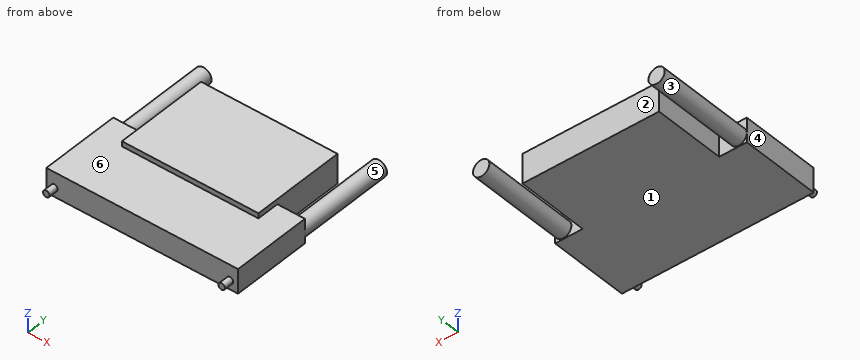
```python
from build123d import *

# Parameters (mm, degrees)
F0_W     = 41.8
F0_H     = 22
F1_DEPTH = 7.45
F2_W     = 41.8
F2_H     = 28.9
F3_DEPTH = 1.55
F4_R     = 1
F5_DEPTH = 3
F6_R     = 2.5
F7_DEPTH = 30


with BuildPart() as f1:
    # F0 (on Top) → F1 (new body)
    with BuildSketch(Plane.XY):
        Polygon((-29.35, 0), (29.35, 0), (29.35, 24.44), (20.9, 24.44), (-20.9, 24.44), (-29.35, 24.44), align=None)
        with Locations((0, 35.44)):
            Rectangle(F0_W, F0_H)
    extrude(amount=F1_DEPTH)

    # F2 (on face) → F3 (join)
    with BuildSketch(Plane.XY.offset(7.45)):
        with Locations((0, 31.99)):
            Rectangle(F2_W, F2_H)
    extrude(amount=F3_DEPTH)

    # F4 (on face) → F5 (join)
    with BuildSketch(Plane.XZ):
        with Locations((-26.85, 2.78)):
            Circle(F4_R)
        with Locations((26.85, 2.78)):
            Circle(F4_R)
    extrude(amount=F5_DEPTH)

    # F6 (on face) → F7 (join)
    with BuildSketch(Plane(origin=(0, 24.44, 0), x_dir=(-1, 0, 0), z_dir=(0, 1, 0))):
        with Locations((-26.85, 2.78)):
            Circle(F6_R)
        with Locations((26.85, 2.78)):
            Circle(F6_R)
    extrude(amount=F7_DEPTH)


solid = f1.part
```
Model file for the job. Use its own axes, mm. Face numbers are marked on the shaded views. A direction names the side the tool comes from. Coordinates: 2 decimals unless noted, no trailing zeros. Order: outer loops, then holes, each group sorted by start corner. A loop starts at its lowest first (then second) coordinate and runs counter-clockwise, first axis right, second up. Notation, with made-up numbers: (55.5, 2.25) -> (93.5, 2.25) arc R19 cw to (93.5, 14.25) -> close; hole circle Ø10 at (-6, 88). An arc over 180 degrees is marked (long way). Answer as a JSON object with one key per item and string values. Group by question number.
1) Which spindle directions (+Z, -Z, +X, -X, +Y, -Y) get a long thin tool onto all of the face, cutting with end or side? Do the marked faces 1, 2 and 3. Say none if no direction does.
2) Cut at B-B, the plane x = 26.85. Write the cut outline in (y, z).
3) Cut at D-D, the plane x = -15.5. Write the cut outline in (y, z), then the cut area to 3 significant figures.
4) Cut at C-C, the plane y = 23. Write the cut outline in (x, z), then the cut area to 3 significant figures.
5) Flat gauge pins, fed straight in: pin 1 (4 mm diameter, centred on y = 33.5, z = 5, fed in from -X); pin 2 (5 mm diameter, centred on x = -8.5, z = 2, fed in from +Y); pin 3 (1.7 mm diameter, centred on x = 3.5, z = 8, fed in from -Y). Where does each tip first touch, or does it go through?
6) Drill centre lines: L1, parallel to X at y = 44.5, z = 2.5; L2, parallel to Z at x = -13, y = 12.5; L3, parallel to Y at x = -11, z = 8. Where is each one in solid material? Low to high.
7) Pull direction X, two halves, no side cores. Call the marked faces 4, 5 and 6: +X half, -X half, draft (parallel to the pull), parting line (faces both ways), or undercut.
8) Cut at A-A, the plane y = 32.5. Write the cut outline in (x, z).
Check values:
{
 "1": {"face 1": "-Z, +X, -X, +Y, -Y", "face 2": "+Z, -Z, +Y", "face 3": "+Y"},
 "2": {"outline": "(-3, 1.78) -> (0, 1.78) -> (0, 0) -> (24.44, 0) -> (24.44, 0.28) -> (54.44, 0.28) -> (54.44, 5.28) -> (24.44, 5.28) -> (24.44, 7.45) -> (0, 7.45) -> (0, 3.78) -> (-3, 3.78) -> close"},
 "3": {"outline": "(0, 0) -> (46.44, 0) -> (46.44, 9) -> (17.54, 9) -> (17.54, 7.45) -> (0, 7.45) -> close", "area": "391 mm²"},
 "4": {"outline": "(-29.35, 0) -> (29.35, 0) -> (29.35, 7.45) -> (20.9, 7.45) -> (20.9, 9) -> (-20.9, 9) -> (-20.9, 7.45) -> (-29.35, 7.45) -> close", "area": "502 mm²"},
 "5": {"pin 1": "stops at x = -29.34", "pin 2": "stops at y = 46.44", "pin 3": "stops at y = 0"},
 "6": {"L1": "x = -29.33 to -24.37, -20.9 to 20.9, 24.37 to 29.33", "L2": "z = 0 to 7.45", "L3": "y = 17.54 to 46.44"},
 "7": {"face 4": "-X half", "face 5": "undercut", "face 6": "draft"},
 "8": {"outline": "circle Ø5 at (-26.85, 2.78); (-20.9, 0) -> (20.9, 0) -> (20.9, 9) -> (-20.9, 9) -> close; circle Ø5 at (26.85, 2.78)"}
}
